from build123d import *

# Parameters (mm, degrees)
SKETCH1_R           = 38.25
BOSS_EXTRUDE1_DEPTH = 250
CUT_EXTRUDE2_DEPTH  = 50


with BuildPart() as part:
    # Sketch1 → Boss-Extrude1 (new body)
    with BuildSketch(Plane.XY):
        Circle(SKETCH1_R)
    boss_extrude1 = extrude(amount=BOSS_EXTRUDE1_DEPTH)

    # Sketch3 → Cut-Extrude2 (cut)
    with BuildSketch(Plane.XY.offset(250)):
        with BuildLine():
            Line((-8.5, 26.940907557), (-8.5, 33.25))
            Line((-8.5, 33.25), (8.5, 33.25))
            Line((8.5, 33.25), (8.5, 26.940907557))
            ThreePointArc((8.5, 26.940907557), (0, -28.25), (-8.5, 26.940907557))
        make_face()
    cut_extrude2 = extrude(amount=-CUT_EXTRUDE2_DEPTH, mode=Mode.SUBTRACT)

    # Mirror1: Boss-Extrude1, Cut-Extrude2 across plane
    add(boss_extrude1.mirror(Plane.XY))
    add(cut_extrude2.mirror(Plane.XY), mode=Mode.SUBTRACT)


solid = part.part
Here's how the part is built. I have some questions about the finished solid (model axes, mm). A direction names the side the tool comes from. Round coordinates to 2 decimals unless told otherwise and drop trailing zeros. Order: outer loops, then holes, each group sorted by start corner. A loop starts at its lowest first (then second) coordinate and runs counter-clockwise, first axis right, second up. Notation, with made-up numbers: (25, 79.5) -> (73, 79.5) arc R23 ccw to (73, 97.5) -> close; hole circle Ø5 at (76, -2). An arc over 180 degrees is marked (long way). Return JSON: item names as keys, results as strings.
Q1. If we mould it in two halves opening along Y, with no side actions, what happens to faces 4 (the cylindrical face through (-30.354, -23.275, 3.5)), 5 (the flat face through (-23, -17, -250)), 6 (the cylindrical face through (1.121, -28.228, -225.35))? For each: released by +Y, released by -Y, zero draft, split by the parting line, or undercut.
Filled sheet:
{"face 4": "split by the parting line", "face 5": "zero draft", "face 6": "undercut"}
Q2. If we section it at A-A on x = 0: List the corners of the cut face in (y, z) for me.
Filled sheet:
{"outline": "(-38.25, -250) -> (-28.25, -250) -> (-28.25, -200) -> (33.25, -200) -> (33.25, -250) -> (38.25, -250) -> (38.25, 250) -> (33.25, 250) -> (33.25, 200) -> (-28.25, 200) -> (-28.25, 250) -> (-38.25, 250) -> close"}
Q3. If we section it at B-B on y = 0: List the corners of the cut face in (x, z) for me, plus the area to 3 significant figures.
Filled sheet:
{"outline": "(-38.25, -250) -> (-28.25, -250) -> (-28.25, -200) -> (28.25, -200) -> (28.25, -250) -> (38.25, -250) -> (38.25, 250) -> (28.25, 250) -> (28.25, 200) -> (-28.25, 200) -> (-28.25, 250) -> (-38.25, 250) -> close", "area": "32,600 mm^2"}
Q4. For pin 1 Ø6 at (x, z) = (9, -60) entering from -Y; pin 2 Ø5 at (x, z) = (23.5, -64) entering from +Y; pin 3 Ø7 at (y, z) = (31.5, -223.5) entering from -X, each with a flat end and sliding along its axis, tell me the tip position at first contact or that it passes through.
Filled sheet:
{"pin 1": "stops at y = -37.78", "pin 2": "stops at y = 31.97", "pin 3": "stops at x = -26.06"}
Q5. I need wall thicknesses on line 1 along Y through (x, z) = (0, 231); line 2 along Z through (x, y) = (11.5, -6.5); line 3 along Y through (x, z) = (31.5, -184). Which ranges of each line are inside material? Lowest first, please. Write a range as from..to.
Filled sheet:
{"line 1": "y = -38.25..-28.25, 33.25..38.25", "line 2": "z = -200..200", "line 3": "y = -21.7..21.7"}
Q6. If we section it at C-C on z = 142: List the corners of the cut face in (x, y) for me, plus the area to 3 significant figures.
Filled sheet:
{"outline": "circle Ø76.5 at (0, 0)", "area": "4,600 mm^2"}
Q7. Which directions (+Z, -Z, +X, -X, +Y, -Y) give clear straight access to the entire face, cutting with the end or side of a thin tool? Please do faces 1 (the flat face through (0, 3, -200)), 2 (the cylindrical face through (1.121, -28.228, 225.35)), 3 (the flat face through (-23, -17, 250)).
Filled sheet:
{"face 1": "-Z", "face 2": "+Z", "face 3": "+Z, +X, -X, +Y, -Y"}
